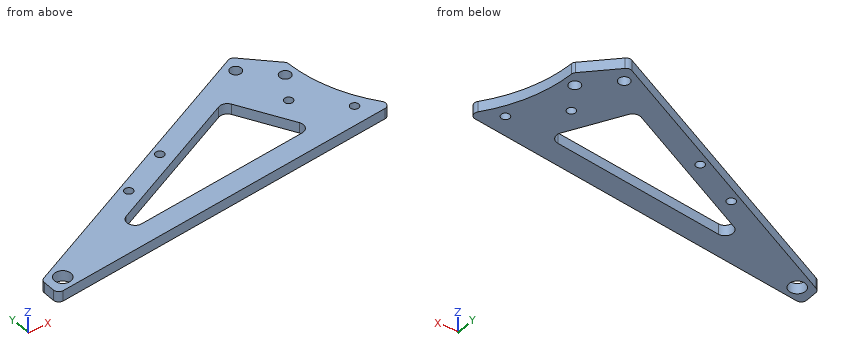
from build123d import *

# Parameters (mm, degrees)
SKETCH_1_R          = 3.1
SKETCH_1_R_2        = 2.1
SKETCH_1_R_3        = 1.6
EXTRUDE_1_DEPTH     = 4
FILLET_2_R          = 2
SKETCH_2_R          = 1.6
CUT_EXTRUDE_1_DEPTH = 20
CUT_EXTRUDE_2_DEPTH = 10
FILLET_3_R          = 3


with BuildPart() as part:
    # 草图1 → 凸台-拉伸1 (new body)
    with BuildSketch(Plane.XY):
        with BuildLine():
            Line((25.982574674, -47.286360788), (-110, -59.293842397))
            Line((-110, -59.293842397), (-110, -51.293842397))
            Line((-110, -51.293842397), (0, 0))
            Line((0, 0), (12.161955086, -12.161955086))
            ThreePointArc((12.161955086, -12.161955086), (15.964760057, -30.946887294), (25.982574674, -47.286360788))
        make_face()
        with Locations((-104, -53.81375969)):
            Circle(SKETCH_1_R, mode=Mode.SUBTRACT)
        with Locations((-2.485281374, -6)):
            Circle(SKETCH_1_R_2, mode=Mode.SUBTRACT)
        with Locations((8.121320344, -16.606601718)):
            Circle(SKETCH_1_R_2, mode=Mode.SUBTRACT)
        with Locations((1.544155877, -27)):
            Circle(SKETCH_1_R_3, mode=Mode.SUBTRACT)
        with Locations((15.686291501, -41.142135624)):
            Circle(SKETCH_1_R_3, mode=Mode.SUBTRACT)
    extrude(amount=EXTRUDE_1_DEPTH)

    # 圆角2
    fillet_2_edges = [part.edges().sort_by_distance(p)[0] for p in [
        (12.161955086, -12.161955086, 2),
        (25.982574674, -47.286360788, 2),
        (-110, -59.293842397, 2),
        (-110, -51.293842397, 2),
        (0, 0, 2),
    ]]
    fillet(fillet_2_edges, radius=FILLET_2_R)

    # 草图2 → 切除-拉伸1 (cut)
    with BuildSketch(Plane.XY.offset(4)):
        with Locations((-45, -24.293978374)):
            Circle(SKETCH_2_R)
        with Locations((-63.126155741, -32.746343609)):
            Circle(SKETCH_2_R)
    extrude(amount=-CUT_EXTRUDE_1_DEPTH, mode=Mode.SUBTRACT)

    # 草图3 → 切除-拉伸2 (cut)
    with BuildSketch(Plane.XY.offset(4)):
        Polygon((-14.605360146, -15.637614638), (-86.566111127, -49.193463907), (-0.110692732, -41.559310422), align=None)
    extrude(amount=-CUT_EXTRUDE_2_DEPTH, mode=Mode.SUBTRACT)

    # 圆角3
    fillet_3_edges = [part.edges().sort_by_distance(p)[0] for p in [
        (-14.605360146, -15.637614638, 2),
        (-0.110692732, -41.559310422, 2),
        (-86.566111127, -49.193463907, 2),
    ]]
    fillet(fillet_3_edges, radius=FILLET_3_R)


solid = part.part
Model file for the job. Use its own axes, mm. Give positions to 0.01 mm unless a question says otherwise; leave off trailing zeros. Order: outer loops, then holes, each group sorted by start corner. A loop starts at its lowest first (then second) coordinate and runs counter-clockwise, first axis right, second up. Notation, with made-up numbers: M 88,84 L 123,84 A13 cw 123,102 Z; hole C 36.5,43 d3. An arc over 180 degrees is marked long. Put each result on its own line as item: value. Start each with the question number.
(1) Pin check, flat tip, straight feed: pin 1 Ø2.5 at (x, y) = (8.12, -16.61) entering from +Z. Stop position of the tip, or through.
(2) Band-saw the part on D-D on x = -45. Give the cut face in (y, z).
(3) Band-saw the part on C-C on x = -104. Give the cut face in (y, z).
(4) Band-saw the part on A-A on z = 1.5. Count the separate pieces of the cut face and the enclosed holes in it, then the cut area to 3 significant figures.
(5) Drill centre lines: L1, parallel to X at y = -25, z = 3.55; L2, parallel to X at y = -26, z = 1.1; L3, parallel to X at y = -19, z = 1.65. Where is each one in solid material? Low to high. Write a range as [from, to].
(6) Band-saw the part on B-B on y = -6. Give the cut face in (x, z).
Results below:
1. pin 1: passes through
2. outline: M -53.55,0 L -45.52,0 L -45.52,4 L -53.55,4 Z; M -29.81,0 L -25.89,0 L -25.89,4 L -29.81,4 Z; M -22.69,0 L -20.98,0 L -20.98,4 L -22.69,4 Z
3. outline: M -58.76,0 L -56.91,0 L -56.91,4 L -58.76,4 Z; M -50.71,0 L -48.5,0 L -48.5,4 L -50.71,4 Z
4. separate pieces: 1
4. enclosed holes: 8
4. area: 2,630 mm2
5. L1: x = [-53.61, -46.44], [-43.56, -34.68], [-9.37, 14.01]
5. L2: x = [-55.76, -36.83], [-8.81, 0.3], [2.79, 14.28]
5. L3: x = [-40.75, -21.82], [-12.73, 12.76]
6. outline: M -12.87,0 L -4.59,0 L -4.59,4 L -12.87,4 Z; M -0.39,0 L 6,0 L 6,4 L -0.39,4 Z
